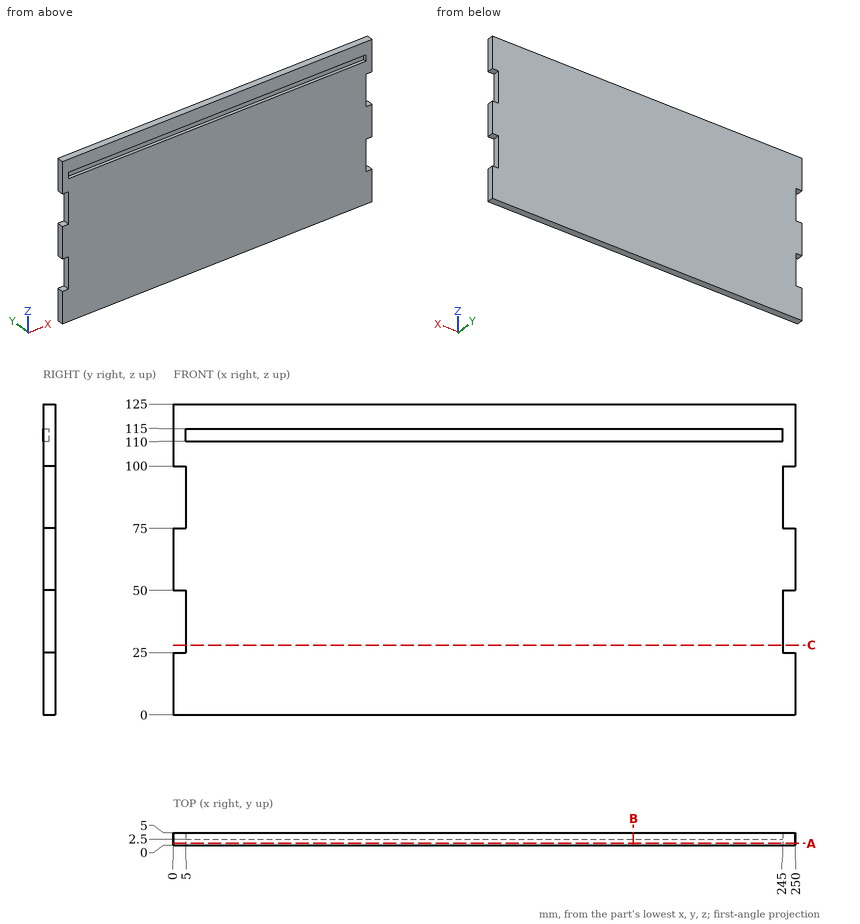
For this review, use the dimensioned drawing (mm, ordinates from the lowest corner) and the shaded views. Give positions to 0.01 mm unless a question says otherwise; leave off trailing zeros. Order: outer loops, then holes, each group sorted by start corner. A loop starts at its lowest first (then second) coordinate and runs counter-clockwise, first axis right, second up.
1) Wall thickness on line 1 (Z direction, x = 92, y = 0.45); line 2 (X direction, y = 0.75, z = 113); line 3 (X direction, y = 2.7, z = 92.5): over which ranges is each line inside the solid? List them lowest first.
2) Take a section at B-B (x = 185). Give the boundary of the cut face in (y, z), then the cut area to 4 significant figures.
3) Take a section at C-C (z = 28). Give the boundary of the cut face in (x, y), then the cut area to 3 significant figures.
4) Insertion check: pin 1 (2.5 mm diameter, centred on y = 2, z = 35, fed in from -X); pin 2 (1.5 mm diameter, centred on y = 3.5, z = 83.5, fed in from +X); pin 3 (2.5 mm diameter, centred on x = 159.5, z = 112, fed in from -Y). Each pin has a flat end and moves straight along its axis. Give the tip position at first contact, or say it passes through.
5) Take a section at A-A (y = 0.75). Give the boundary of the cut face in (x, z), then the cut area to 4 significant figures.
Derived:
1. line 1: z = 0 to 110, 115 to 125
1. line 2: x = 0 to 5, 245 to 250
1. line 3: x = 5 to 245
2. outline: (0, 0) - (5, 0) - (5, 125) - (0, 125) - (0, 115) - (2.5, 115) - (2.5, 110) - (0, 110) - close
2. area: 612.5 mm2
3. outline: (5, 0) - (245, 0) - (245, 5) - (5, 5) - close
3. area: 1,200 mm2
4. pin 1: stops at x = 5
4. pin 2: stops at x = 245
4. pin 3: stops at y = 2.5
5. outline: (0, 0) - (250, 0) - (250, 25) - (245, 25) - (245, 50) - (250, 50) - (250, 75) - (245, 75) - (245, 100) - (250, 100) - (250, 125) - (0, 125) - (0, 100) - (5, 100) - (5, 75) - (0, 75) - (0, 50) - (5, 50) - (5, 25) - (0, 25) - close; hole (5, 110) - (245, 110) - (245, 115) - (5, 115) - close
5. area: 29,550 mm2
